```python
from build123d import *

# Parameters (mm, degrees)
F2_DEPTH = 7.14375
F0_R     = 5.55625
F3_DEPTH = 50.8
F5_SIZE  = 0.762


# Not quite as in the source:
# - a length typed as a fraction of an inch, garbled in the dataset ("3 / 203.2 mm" for 3/8 in), is restored


with BuildPart() as f2:
    # F1 (on Top) → F2 (new body)
    with BuildSketch(Plane.XY):
        Polygon((7.9375, 4.5827177617), (0, 9.1654355234), (-7.9375, 4.5827177617), (-7.9375, -4.5827177617), (0, -9.1654355234), (7.9375, -4.5827177617), align=None)
    extrude(amount=F2_DEPTH)

    # F0 (on Top) → F3 (join)
    with BuildSketch(Plane.XY):
        Circle(F0_R)
    extrude(amount=F3_DEPTH)

    # F5
    f5_edges = [f2.edges().sort_by_distance(p)[0] for p in [
        (-5.55625, 0, 50.8),
    ]]
    chamfer(f5_edges, length=F5_SIZE)


solid = f2.part
```
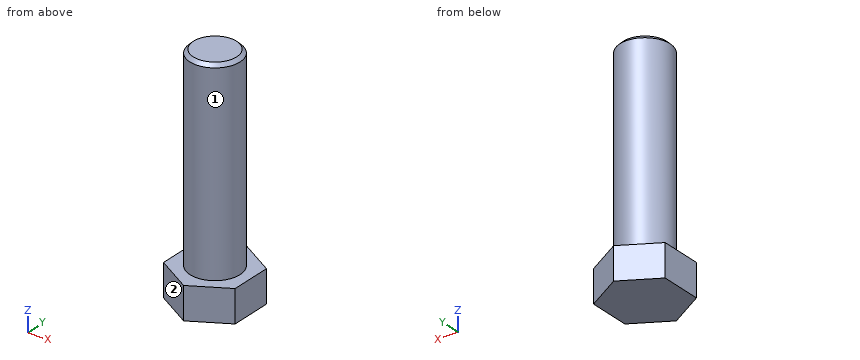
For this review, take the finished solid that the model builds, in its own axes (mm). Face numbers are marked on the shaded views. A direction names the side the tool comes from. Round coordinates to 2 decimals unless told otherwise and drop trailing zeros. Loops run counter-clockwise (first coordinate to the right, second up) from the corner with the lowest first, then second, coordinate; pieces in that order, holes last.
(1) Clearance check with flat-ended pins moving along their axes: P1, Ø1, axis at x = 3, z = 13, coming from the +Y side; P2, Ø8, axis at x = 6, z = 41, coming from the -Y side; P3, Ø1.5, axis at y = -1, z = 37.5, coming from the -X side. State where each tip first meets the part, or that it passes through.
Returned:
P1: stops at y = 4.96
P2: stops at y = -5.18
P3: stops at x = -5.55
(2) We need section A-A (y = 0). Give the boundary of the cut face in (x, z).
Returned:
outline: (-7.94, 0) - (7.94, 0) - (7.94, 7.14) - (5.56, 7.14) - (5.56, 50.04) - (4.79, 50.8) - (-4.79, 50.8) - (-5.56, 50.04) - (-5.56, 7.14) - (-7.94, 7.14) - close
(3) Wall thickness on line 1 along Z through (x, y) = (-3.25, -5); line 2 along X through (y, z) = (-2, 40); line 3 along Y through (x, z) = (3.75, 35): over which ranges is each line inside the solid? List them lowest first.
Returned:
line 1: z = 0 to 7.14
line 2: x = -5.18 to 5.18
line 3: y = -4.1 to 4.1
(4) Tool access review of the marked faces 1 and 2: name each direction out of +Z, -Z, +X, -X, +Y, -Y from which nothing blocks a thin tool from reaching the whole face with its end or side.
Returned:
face 1: +Z
face 2: +Z, -Z, -X, -Y
